Design review of the part built by this model. Coordinates are the model's own, in mm. A direction names the side the tool comes from. Coordinates: 2 decimals unless noted, no trailing zeros. Loops run counter-clockwise (first coordinate to the right, second up) from the corner with the lowest first, then second, coordinate; pieces in that order, holes last. Notation, with made-up numbers: (71.25, -27) -> (120.25, -27) arc R27 ccw to (120.25, 7) -> close; hole circle Ø11 at (31.5, -5). An arc over 180 degrees is marked (long way). Answer in a Markdown table with one row per item.
```python
from build123d import *

# Parameters (mm, degrees)
BOSS_EXTRUDE2_DEPTH = 25.4
SKETCH2_R           = 15.5575
CUT_EXTRUDE1_DEPTH  = 49.568160867


with BuildPart() as part:
    # Sketch1 → Boss-Extrude2 (new body)
    with BuildSketch(Plane.XY):
        Polygon((-34.925, -22.225), (34.925, -22.225), (34.925, -15.875), (22.225, -15.875), (22.225, 22.225), (-22.225, 22.225), (-22.225, -15.875), (-34.925, -15.875), align=None)
    extrude(amount=BOSS_EXTRUDE2_DEPTH)

    # Sketch2 → Cut-Extrude1 (cut, through all)
    with BuildSketch(Plane(origin=(0, 0, 0), x_dir=(-1, 0, 0), z_dir=(0, 0, -1))):
        Circle(SKETCH2_R)
    extrude(amount=-CUT_EXTRUDE1_DEPTH, mode=Mode.SUBTRACT)


solid = part.part
```
(1) Tool access review of faces 1 (the flat face through (22.225, 3, 13)), 2 (the flat face through (-22.225, 3, 13)), 3 (the flat face through (-34.925, -19, 13)): name each direction out of +Z, -Z, +X, -X, +Y, -Y from which nothing blocks a thin tool from reaching the whole face with its end or side.
Evaluation:
| item | result |
|---|---|
| face 1 | +Z, -Z, +X, +Y |
| face 2 | +Z, -Z, -X, +Y |
| face 3 | +Z, -Z, -X, +Y, -Y |
(2) Take a section at A-A on x = 0. Give the boundary of the cut face in (y, z) (1 decimal), and give its area (3 significant figures).
Evaluation:
| item | result |
|---|---|
| outline | (-22.2, 0) -> (-15.6, 0) -> (-15.6, 25.4) -> (-22.2, 25.4) -> close; (15.6, 0) -> (22.2, 0) -> (22.2, 25.4) -> (15.6, 25.4) -> close |
| area | 339 mm² |
(3) To check wall thickness, follow probe 1 along Y at (x, z) = (0, 5) (1 decimal); probe 2 along X at (y, z) = (16.5, 19.5) (3 decimals); probe 3 along X at (y, z) = (4, 7.5) (3 decimals). State the ranges of each line that lie inside material, in increasing order.
Evaluation:
| item | result |
|---|---|
| probe 1 | y = -22.2 to -15.6, 15.6 to 22.2 |
| probe 2 | x = -22.225 to 22.225 |
| probe 3 | x = -22.225 to -15.034, 15.034 to 22.225 |
(4) Take a section at B-B on z = 16.5. Give the boundary of the cut face in (x, y) (1 decimal).
Evaluation:
| item | result |
|---|---|
| outline | (-34.9, -22.2) -> (34.9, -22.2) -> (34.9, -15.9) -> (22.2, -15.9) -> (22.2, 22.2) -> (-22.2, 22.2) -> (-22.2, -15.9) -> (-34.9, -15.9) -> close; hole circle Ø31.1 at (0, 0) |
(5) For pin 1 (10 mm diameter, centred on y = -10.5, z = 16.5, fed in from +X) (3 decimals); pin 2 (4 mm diameter, centred on x = -30.5, z = 16.5, fed in from +Y) (3 decimals); pin 3 (14 mm diameter, centred on x = 28, z = 12.5, fed in from +Y) (3 decimals); pin 4 (7.5 mm diameter, centred on y = 1, z = 14, fed in from -X) (3 decimals), all flat-tipped, find the tip position at first contact; note any pin that passes through.
Evaluation:
| item | result |
|---|---|
| pin 1 | stops at x = 22.225 |
| pin 2 | stops at y = -15.875 |
| pin 3 | stops at y = 22.225 |
| pin 4 | stops at x = -22.225 |
(6) Take a section at D-D on x = 26.5. Give the boundary of the cut face in (y, z) (3 decimals), and give its area (3 significant figures).
Evaluation:
| item | result |
|---|---|
| outline | (-22.225, 0) -> (-15.875, 0) -> (-15.875, 25.4) -> (-22.225, 25.4) -> close |
| area | 161 mm² |
(7) Draft analysis for pull direction Y (two halves, no side actions). For faces 4 (the flat face through (0, -22.225, 13)), 5 (the flat face through (-8, -15, 0)), 6 (the cylindrical face through (3.37, -15.19, 12.52)), 7 (the flat face through (-28, -15.875, 13)), state which applies: pulls with the +Y half, pulls with the -Y half, needs draft (parallel to the pull), parting line crosses it, or undercut.
Evaluation:
| item | result |
|---|---|
| face 4 | pulls with the -Y half |
| face 5 | needs draft |
| face 6 | undercut |
| face 7 | pulls with the +Y half |
